Check sheet for the drawn part. Datum: minimum x, y, z corner. Units: mm. A direction names the side the tool comes from. Give positions to 0.01 mm unless a question says otherwise; leave off trailing zeros. Loops run counter-clockwise (first coordinate to the right, second up) from the corner with the lowest first, then second, coordinate; pieces in that order, holes last. Notation, with made-up numbers: (22.5, 6.5) -> (45.5, 6.5) arc R23 ccw to (45.5, 33.5) -> close; hole circle Ø1 at (54, -17.5). An arc over 180 degrees is marked (long way). One line per question, with ' | ' between items.
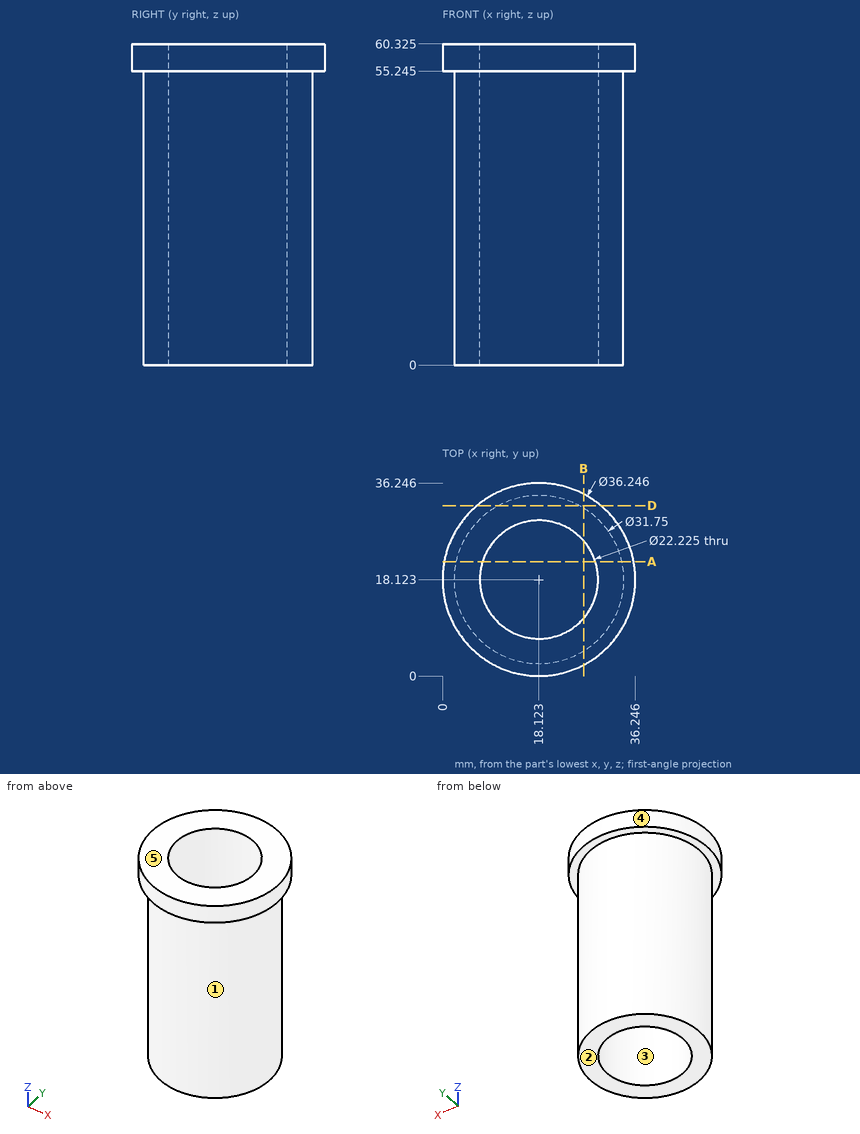
Item 1: Release check for a two-part mould opening along X. For the marked faces 3, 4 and 5 record: pulls with the +X half, pulls with the -X half, needs draft (parallel to the pull), parting line crosses it, or undercut.
Result:
face 3: undercut | face 4: parting line crosses it | face 5: needs draft
Item 2: Sectioned sample at D-D (y = 32). Record the cut outline in (x, z) (1 decimal).
Result:
outline: (6.5, 55.2) -> (10.4, 55.2) -> (10.4, 0) -> (25.8, 0) -> (25.8, 55.2) -> (29.8, 55.2) -> (29.8, 60.3) -> (6.5, 60.3) -> close
Item 3: Depth check by flat-ended pin: pin 1 Ø4 at (y, z) = (11.5, 18) entering from +X; pin 2 Ø1.5 at (x, z) = (8.5, 15.5) entering from +Y; pin 3 Ø13.5 at (x, y) = (18.12, 18.12) entering from -Z; pin 4 Ø5 at (x, z) = (6.5, 39.5) entering from -Y. Enter the tip coordinate at first touch or a pass-through.
Result:
pin 1: x = 33.31 | pin 2: y = 31.29 | pin 3: through | pin 4: y = 5.13
Item 4: Scan lines: probe 1 along Z at (x, y) = (25, 34.5) (3 decimals); probe 2 along Y at (x, z) = (20, 28.5); probe 3 along X at (y, z) = (19, 11) (1 decimal). Record each from-to range of solid material in increasing order.
Result:
probe 1: 55.245 to 60.325 | probe 2: 2.36 to 7.17, 29.08 to 33.89 | probe 3: 2.3 to 7, 29.2 to 34
Item 5: Sectioned sample at B-B (x = 26.5). Record the cut outline in (y, z) (1 decimal).
Result:
outline: (2.1, 55.2) -> (4.6, 55.2) -> (4.6, 0) -> (10.8, 0) -> (10.8, 60.3) -> (2.1, 60.3) -> close; (25.4, 0) -> (31.6, 0) -> (31.6, 55.2) -> (34.2, 55.2) -> (34.2, 60.3) -> (25.4, 60.3) -> close
Item 6: Sectioned sample at A-A (y = 21.5). Record the cut outline in (x, z) (1 decimal).
Result:
outline: (0.3, 55.2) -> (2.6, 55.2) -> (2.6, 0) -> (7.5, 0) -> (7.5, 60.3) -> (0.3, 60.3) -> close; (28.7, 0) -> (33.6, 0) -> (33.6, 55.2) -> (35.9, 55.2) -> (35.9, 60.3) -> (28.7, 60.3) -> close
Item 7: Set-up check for the marked faces 1 and 2: record each of +Z, -Z, +X, -X, +Y, -Y from which the full face is reachable in a straight line by a thin tool's end or side.
Result:
face 1: -Z | face 2: -Z, +X, -X, +Y, -Y
